For this review, take the finished solid that the model builds, in its own axes (mm). A direction names the side the tool comes from. Give positions to 0.01 mm unless a question says otherwise; leave off trailing zeros. Write each loop counter-clockwise with the first axis right and the second up, starting at its lowest first coordinate (ties: lowest second). Pieces come first, ordered by that corner, then holes. Notation, with made-up numbers: M -31.75,16.25 L -27.75,16.25 A19 ccw -27.75,43.25 Z; hole C -34,84.5 d2. An arc over 180 degrees is marked long. One line per item, written item: value. Start each with the question number.
Item 1: To check wall thickness, follow probe 1 along Z at (x, y) = (5, 7); probe 2 along Z at (x, y) = (-4, -6.5); probe 3 along Y at (x, z) = (0, -12.1). State the ranges of each line that lie inside material, in increasing order.
Item 2: Consider section A-A, the plane z = -18.5. Write out the cut boundary in (x, y).
Item 3: Consider section B-B, the plane y = 0. Give the number of separate pieces and of enclosed holes in the cut face, and give its area (3 significant figures).
Item 4: Clearance check with flat-ended pins moving along their axes: pin 1 Ø6 at (x, z) = (5, -7.5) entering from -Y; pin 2 Ø0.6 at (x, z) = (1.5, -11.5) entering from +Y; pin 3 Ø4 at (x, z) = (-5, -5.5) entering from -Y. State where each tip first meets the part, or that it passes through.
Item 5: Tool access review of faces 1 (the face through (0, -3, -16.25)), 2 (the face through (2, 2, -13.75)), 3 (the face through (2.4, -1.8, -21.4)), 4 (the face through (-0.54, -2.44, -13)), 5 (the face through (6.25, -1.33, -22.36)): name each direction out of +Z, -Z, +X, -X, +Y, -Y from which nothing blocks a thin tool from reaching the whole face with its end or side.
Item 6: Mouldability with a two-part tool opening along Y and no side actions: class faces 6 (the face through (-1.84, 1.69, -4.56)), 7 (the face through (-2, 2, -11.25)), 8 (the face through (-8, -6, -13)) as released by +Y, released by -Y, zero draft, split by the parting line, or undercut.
```python
from build123d import *

# Parameters (mm, degrees)
SKETCH_1_R               = 10
SKETCH_1_R_2             = 2.5
EXTRUDE_1_DEPTH          = 26
SKETCH_2_R               = 1.5
SKETCH_2_W               = 0.5
SKETCH_2_H               = 15
CUT_EXTRUDE_1_DEPTH      = 11
CUT_EXTRUDE_1_DEPTH_BACK = 11
SKETCH_3_R               = 3
CUT_EXTRUDE_2_DEPTH      = 9.25
FILLET_1_R               = 1


with BuildPart() as part:
    # Эскиз1 → Бобышка-Вытянуть1 (new body)
    with BuildSketch(Plane.XY):
        Circle(SKETCH_1_R)
        Circle(SKETCH_1_R_2, mode=Mode.SUBTRACT)
    extrude(amount=-EXTRUDE_1_DEPTH)

    # Эскиз2 → Вырез-Вытянуть1 (cut, two sides)
    with BuildSketch(Plane(origin=(0, 0, 0), x_dir=(0, 0, -1), z_dir=(1, 0, 0))) as cut_extrude_1_sk:
        with Locations((4.333333333, 0)):
            Circle(SKETCH_2_R)
        with Locations((21.666666667, 0)):
            Circle(SKETCH_2_R)
        with Locations((13.5, 2.5)):
            Rectangle(SKETCH_2_W, SKETCH_2_H)
        with Locations((15.5, 2.5)):
            Rectangle(SKETCH_2_W, SKETCH_2_H)
        with Locations((14.5, -2.5)):
            Rectangle(SKETCH_2_W, SKETCH_2_H)
        with Locations((16.5, -2.5)):
            Rectangle(SKETCH_2_W, SKETCH_2_H)
        with Locations((11.5, 2.5)):
            Rectangle(SKETCH_2_W, SKETCH_2_H)
        with Locations((12.5, -2.5)):
            Rectangle(SKETCH_2_W, SKETCH_2_H)
        with Locations((9.5, 2.5)):
            Rectangle(SKETCH_2_W, SKETCH_2_H)
        with Locations((10.5, -2.5)):
            Rectangle(SKETCH_2_W, SKETCH_2_H)
    extrude(amount=CUT_EXTRUDE_1_DEPTH, mode=Mode.SUBTRACT)
    extrude(cut_extrude_1_sk.sketch, amount=-CUT_EXTRUDE_1_DEPTH_BACK, mode=Mode.SUBTRACT)

    # Эскиз3 → Вырез-Вытянуть2 (cut)
    with BuildSketch(Plane(origin=(0, 0, -26), x_dir=(-1, 0, 0), z_dir=(0, 0, -1))):
        Circle(SKETCH_3_R)
    extrude(amount=-CUT_EXTRUDE_2_DEPTH, mode=Mode.SUBTRACT)

    # Скругление1
    fillet_1_edges = [part.edges().sort_by_distance(p)[0] for p in [
        (-10, 0, 0),
        (-10, 0, -26),
    ]]
    fillet(fillet_1_edges, radius=FILLET_1_R)


solid = part.part
```
Model answer:
1. probe 1: z = -26 to -15.75, -15.25 to -13.75, -13.25 to -11.75, -11.25 to -9.75, -9.25 to 0
1. probe 2: z = -26 to -16.75, -16.25 to -14.75, -14.25 to -12.75, -12.25 to -10.75, -10.25 to 0
1. probe 3: y = -10 to -2.5, 2.5 to 10
2. outline: C 0,0 d20; hole C 0,0 d6
3. separate pieces: 22
3. enclosed holes: 0
3. area: 233 mm2
4. pin 1: stops at y = -9.8
4. pin 2: stops at y = 9.91
4. pin 3: stops at y = -9.54
5. face 1: +X, -X, -Y
5. face 2: +X, -X, +Y
5. face 3: -Z
5. face 4: +Z, -Z
5. face 5: +X, -X
6. face 6: undercut
6. face 7: zero draft
6. face 8: split by the parting line
